```python
from build123d import *

# Parameters (mm, degrees)
F0_W      = 70
F0_H      = 70
F0_W_2    = 60
F0_H_2    = 60
F1_DEPTH  = 3
F2_W      = 70
F2_H      = 70
F2_W_2    = 60
F2_H_2    = 60
F3_DEPTH  = 40
F4_W      = 50
F4_H      = 20
F5_DEPTH  = 71
F6_W      = 50
F6_H      = 20
F7_DEPTH  = 70
F11_R     = 1.6
F12_DEPTH = 25


with BuildPart() as f1:
    # F0 (on Top) → F1 (new body)
    with BuildSketch(Plane.XY):
        Rectangle(F0_W, F0_H)
        Rectangle(F0_W_2, F0_H_2, mode=Mode.SUBTRACT)
        Rectangle(F0_W_2, F0_H_2)
    extrude(amount=F1_DEPTH)

    # F2 (on face) → F3 (join)
    with BuildSketch(Plane.XY.offset(3)):
        Rectangle(F2_W, F2_H)
        Rectangle(F2_W_2, F2_H_2, mode=Mode.SUBTRACT)
    extrude(amount=F3_DEPTH)

    # F4 (on face) → F5 (cut)
    with BuildSketch(Plane.XZ.offset(35)):
        with Locations((0, 33)):
            Rectangle(F4_W, F4_H)
    extrude(amount=-F5_DEPTH, mode=Mode.SUBTRACT)

    # F6 (on face) → F7 (cut)
    with BuildSketch(Plane.YZ.offset(35)):
        with Locations((0, 33)):
            Rectangle(F6_W, F6_H)
    extrude(amount=-F7_DEPTH, mode=Mode.SUBTRACT)

    # F11 (on offset) → F12 (cut)
    with BuildSketch(Plane.XY.offset(45)):
        with Locations((32.5, 32.5)):
            Circle(F11_R)
        with Locations((32.5, -32.5)):
            Circle(F11_R)
        with Locations((-32.5, 32.5)):
            Circle(F11_R)
        with Locations((-32.5, -32.5)):
            Circle(F11_R)
    extrude(amount=-F12_DEPTH, mode=Mode.SUBTRACT)


solid = f1.part
```
Can you work these out from the model? Positions are in its coordinate system, mm. A direction names the side the tool comes from. Coordinates: 2 decimals unless noted, no trailing zeros. Order: outer loops, then holes, each group sorted by start corner. A loop starts at its lowest first (then second) coordinate and runs counter-clockwise, first axis right, second up. Notation, with made-up numbers: (0.5, 68.25) - (42.5, 68.25) arc R27 cw to (42.5, 99.25) - close; hole circle Ø7 at (35.25, 83). An arc over 180 degrees is marked (long way). Answer in a Markdown table with one row per item.
1. For faces 1 (the flat face through (33, 25, 33)), 2 (the flat face through (0, 32, 23)), 3 (the flat face through (-33, 33, 20)), 4 (the flat face through (31, -31, 43)), which set-ups out of +Z, -Z, +X, -X, +Y, -Y let a thin tool reach every point of the face, with its end or its side?
Reply:
| item | result |
|---|---|
| face 1 | +Z, +X, -X |
| face 2 | +Z, +Y, -Y |
| face 3 | +Z |
| face 4 | +Z, +X, -X, +Y, -Y |
2. Suppose I cut it at B-B (x = -16). Please give me the cut outline in (y, z).
Reply:
| item | result |
|---|---|
| outline | (-35, 0) - (35, 0) - (35, 23) - (30, 23) - (30, 3) - (-30, 3) - (-30, 23) - (-35, 23) - close |
3. For pin 1 (2.5 mm diameter, centred on x = 32.5, y = 32.5, fed in from +Z); pin 2 (2.5 mm diameter, centred on x = -31.5, y = 10.5, fed in from +Z); pin 3 (8 mm diameter, centred on x = 14, y = 22, fed in from +Z), each with a flat end and sliding along its axis, tell me the tip position at first contact or that it passes through.
Reply:
| item | result |
|---|---|
| pin 1 | stops at z = 20 |
| pin 2 | stops at z = 23 |
| pin 3 | stops at z = 3 |
4. Suppose I cut it at D-D (z = 11). Please give me the cut outline in (x, y), and give its area (3 significant figures).
Reply:
| item | result |
|---|---|
| outline | (-35, -35) - (35, -35) - (35, 35) - (-35, 35) - close; hole (-30, -30) - (30, -30) - (30, 30) - (-30, 30) - close |
| area | 1,300 mm^2 |
5. If I drill on line 1 along Y through (x, z) = (32.5, 28); line 2 along Y through (x, z) = (13.5, 9), over which ranges is the centre line in solid material (lowest first)?
Reply:
| item | result |
|---|---|
| line 1 | y = -35 to -34.1, -30.9 to -25, 25 to 30.9, 34.1 to 35 |
| line 2 | y = -35 to -30, 30 to 35 |
6. If we mould it in two halves opening along Y, with no side actions, what happens to faces 5 (the flat face through (0, 35, 16)), 6 (the flat face through (-25, 32, 33)), 7 (the flat face through (0, 0, 3))? For each: pulls with the +Y half, pulls with the -Y half, needs draft (parallel to the pull), parting line crosses it, or undercut.
Reply:
| item | result |
|---|---|
| face 5 | pulls with the +Y half |
| face 6 | needs draft |
| face 7 | undercut |
7. Suppose I cut it at A-A (z = 24.5). Please give me the cut outline in (x, y), and give its area (3 significant figures).
Reply:
| item | result |
|---|---|
| outline | (-35, -35) - (-25, -35) - (-25, -30) - (-30, -30) - (-30, -25) - (-35, -25) - close; (-35, 25) - (-30, 25) - (-30, 30) - (-25, 30) - (-25, 35) - (-35, 35) - close; (25, -35) - (35, -35) - (35, -25) - (30, -25) - (30, -30) - (25, -30) - close; (25, 30) - (30, 30) - (30, 25) - (35, 25) - (35, 35) - (25, 35) - close; hole circle Ø3.2 at (-32.5, -32.5); hole circle Ø3.2 at (-32.5, 32.5); hole circle Ø3.2 at (32.5, -32.5); hole circle Ø3.2 at (32.5, 32.5) |
| area | 268 mm^2 |
8. Suppose I cut it at C-C (y = 32.5). Please give me the cut outline in (x, z), and give its area (3 significant figures).
Reply:
| item | result |
|---|---|
| outline | (-35, 0) - (35, 0) - (35, 43) - (34.1, 43) - (34.1, 20) - (30.9, 20) - (30.9, 43) - (25, 43) - (25, 23) - (-25, 23) - (-25, 43) - (-30.9, 43) - (-30.9, 20) - (-34.1, 20) - (-34.1, 43) - (-35, 43) - close |
| area | 1,860 mm^2 |
